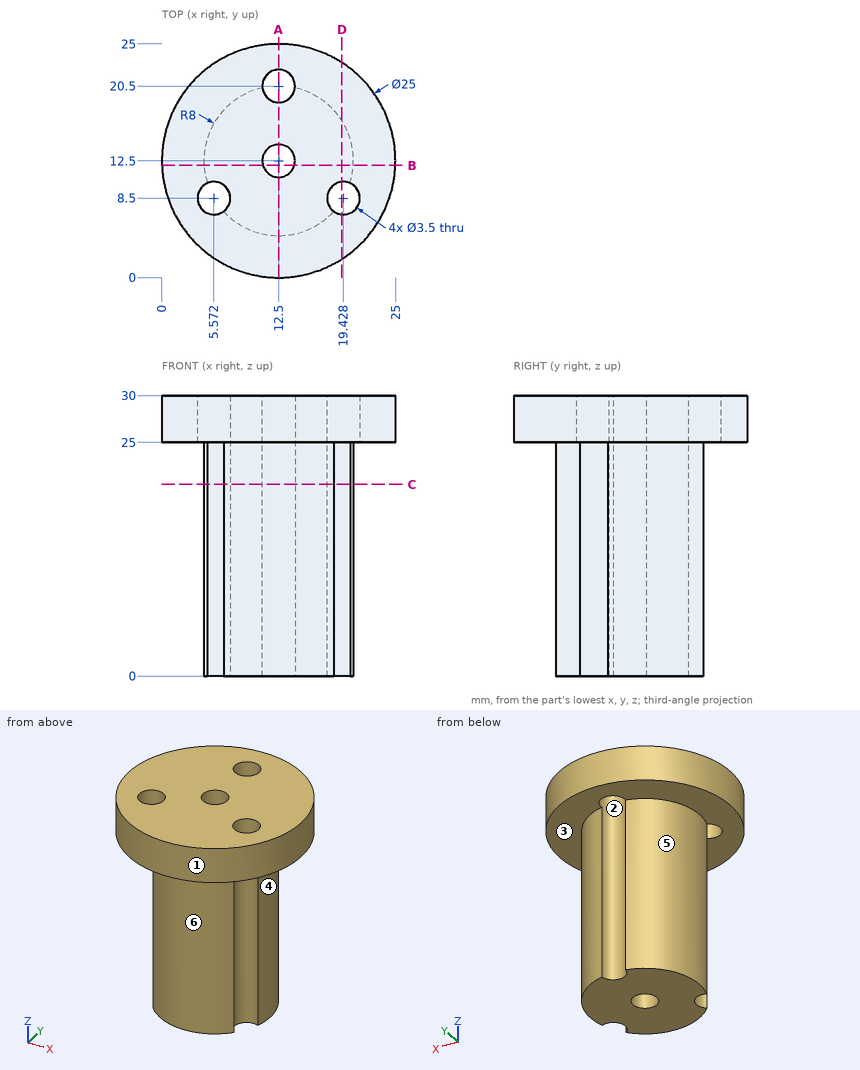
Design review of the part shown in the three views and the two pictorial views. Dimensions are in mm from the part's minimum x, y and z. A direction names the side the tool comes from. Round coordinates to 2 decimals unless told otherwise and drop trailing zeros. Loops run counter-clockwise (first coordinate to the right, second up) from the corner with the lowest first, then second, coordinate; pieces in that order, holes last. Notation, with made-up numbers: M 34.25,18.5 L 44.25,18.5 A8 ccw 44.25,25.5 Z; hole C 60,63.25 d6. An arc over 180 degrees is marked long. Answer as a JSON object with one key per item and string values.
Item 1: Clearance check with flat-ended pins moving along their axes: P1, Ø3, axis at y = 13.5, z = 24.5, coming from the -X side; P2, Ø3, axis at x = 8.5, z = 3.5, coming from the +Y side; P3, Ø1, axis at y = 16, z = 23.5, coming from the -X side; P4, Ø2, axis at x = 7, z = 5.5, coming from the +Y side (1 decimal). State where each tip first meets the part, or that it passes through.
Answer sheet:
{"P1": "stops at x = 0", "P2": "stops at y = 20.1", "P3": "stops at x = 5.08", "P4": "stops at y = 19.1"}
Item 2: We need section A-A on x = 12.5. Give the boundary of the cut face in (y, z), and give its area (3 significant figures).
Answer sheet:
{"outline": "M 0,25 L 4.5,25 L 4.5,0 L 10.75,0 L 10.75,30 L 0,30 Z; M 14.25,0 L 18.75,0 L 18.75,30 L 14.25,30 Z; M 22.25,25 L 25,25 L 25,30 L 22.25,30 Z", "area": "359 mm^2"}
Item 3: We need section C-C on z = 20.5. Give the boundary of the cut face in (x, y).
Answer sheet:
{"outline": "M 4.87,10.1 A1.75 cw 6.61,7.09 A8 ccw 18.39,7.09 A1.75 cw 20.13,10.1 A8 ccw 14.24,20.31 A1.75 cw 10.76,20.31 A8 ccw Z; hole C 12.5,12.5 d3.5"}
Item 4: Machinability: for the marked faces 4, 5 and 6, which of the approach directions +Z, -Z, +X, -X, +Y, -Y give a long, thin tool a straight path to every point of the face, cutting with its end or side? Answer none if there is none.
Answer sheet:
{"face 4": "-Z, +X", "face 5": "-Z, -X", "face 6": "-Z, -Y"}
Item 5: We need section B-B on y = 12. Give the boundary of the cut face in (x, z).
Answer sheet:
{"outline": "M 0.01,25 L 4.52,25 L 4.52,0 L 10.82,0 L 10.82,30 L 0.01,30 Z; M 14.18,0 L 20.48,0 L 20.48,25 L 24.99,25 L 24.99,30 L 14.18,30 Z"}
Item 6: The part is to be moulded in two halves that separate along Y. For the marked faces 1, 2 and 3, say which applies: pulls with the +Y half, pulls with the -Y half, needs draft (parallel to the pull), parting line crosses it, or undercut.
Answer sheet:
{"face 1": "parting line crosses it", "face 2": "undercut", "face 3": "needs draft"}
Item 7: Wall thickness on L1, parallel to Y at x = 12.5, z = 7; L2, parallel to Z at x = 15.75, y = 3; L3, parallel to X at y = 9.25, z = 28.5: over which ranges is each line inside the solid? List them lowest first. Write a range as from..to.
Answer sheet:
{"L1": "y = 4.5..10.75, 14.25..18.75", "L2": "z = 25..30", "L3": "x = 0.43..3.99, 7.15..17.85, 21.01..24.57"}
Item 8: We need section D-D on x = 19.25. Give the boundary of the cut face in (y, z), and give its area (3 significant figures).
Answer sheet:
{"outline": "M 1.98,25 L 6.76,25 L 6.76,30 L 1.98,30 Z; M 10.24,0 L 16.79,0 L 16.79,25 L 23.02,25 L 23.02,30 L 10.24,30 Z", "area": "252 mm^2"}
